Autodesk Inventor part; units mm, degrees
ref_plane "Work Plane1" through (0, 0, 0) normal (0.6427876, -0.7660444, 0) x (0, 0, -1)
ref_plane "Work Plane2" through (0, 14.3, -20) normal (-0.6427876, 0.7660444, 0) x (0, 0, -1)
ref_plane "YZ Plane" through (0, 0, 0) normal (1, 0, 0) x (0, 1, 0)
sketch "Sketch1" plane through (0, 0, 0) normal (0, 1, 0) x (-1, 0, 0)
  circle A0 centre (0, 0) radius 5.075
  circle A1 centre (0, 0) radius 20
  line L0 (1.5, -3.825) -> (-1.5, -3.825)
  line L1 (-1.5, -3.825) -> (-1.5, -6.325)
  line L2 (-1.5, -6.325) -> (1.5, -6.325)
  line L3 (1.5, -6.325) -> (1.5, -3.825)
  line L4 (1.5, -3.825) -> (-1.5, -6.325) construction
  line L5 (-1.5, -3.825) -> (1.5, -6.325) construction
  circle A2 centre (0, 0) radius 2.5
  circle A3 centre (0, 0) radius 8.754
  point P0 (0, -5.075)
  point P1 (-1.5, -4.8483)
  point P2 (1.5, -4.8483)
  dimension "d0" = 10.15
  dimension "d1" = 40
  dimension "d2" = 1.25
  dimension "d3" = 3
  dimension "d17" = 5
extrude "Extrusion1" add sketch "Sketch1" along normal blind 14.3 contours A1 | A3
sketch "Sketch2" plane through (0, 0, 0) normal (1, 0, 0) x (0, 1, 0)
  line L0 (0, 0) -> (14.3, 0)
  line L1 (14.3, 0) -> (14.3, -20)
  line L2 (14.3, -20) -> (0, -20) construction
  line L3 (0, -20) -> (0, 0)
  line L4 (0, -20) -> (14.3, -20) construction
  line L5 (14.3, -20) -> (14.3, -20.0661)
  line L6 (0, -20) -> (14.3, -20)
  circle A0 centre (7.15, -20) radius 2.5
  line L7 (9.65, -20) -> (4.65, -20)
  line L8 (4.65, -20) -> (4.65, -28)
  line L9 (4.65, -28) -> (9.65, -28)
  line L10 (9.65, -28) -> (9.65, -20)
  line L11 (14.3, -20) -> (0, -20)
  line L12 (0, -20) -> (0, -28)
  line L13 (0, -28) -> (14.3, -28)
  line L14 (14.3, -28) -> (14.3, -20)
  point P0 (14.3, -20)
  point P1 (14.3, -20)
  dimension "d22" = 5
  dimension "d7" = 20
  dimension "d10" = 14.3
  dimension "d23" = 8
  dimension "d31" = 8
  dimension "d41" = 14.3
  dimension "d42" = 5
revolve "Revolution1" add sketch "Sketch2" angle 360 about axis through (0, 0, 0) along (0, 1, 0) contours L6 L8 L13 L12 | L5 L14 L13 L10 L6
extrude "Extrusion3" add sketch "Sketch1" against normal blind 2 contours A0 L3 L0 L1 | L1 L0 L3 A0 | A0 L3 L2 L1 | A3
revolve "Revolution4" cut sketch "Sketch2" angle 360 about axis through (0, 0, 0) along (0, 1, 0) picked at (7.2504, -19.1727) contours A0 L6
sketch "Sketch3" plane through (0, 0, 0) normal (0, -1, 0) x (1, 0, 0)
  line L0 (0, 0) -> (0, -22)
  dimension "d25" = 22
ref_plane "Work Plane1" through (0, 0, 0) normal (0.6427876, -0.7660444, 0) x (0, 0, -1)
sketch "Sketch4" plane through (0, 0, 0) normal (0.6427876, -0.7660444, 0) x (0, 0, -1)
  ellipse E0 centre (0, 2.7318) end of major axis (22, 2.7318) minor radius 16.853
  line L0 (0, 0) -> (22, 0)
  circle A0 centre (22, 0) radius 3.75
  dimension "d27" = 22
  dimension "d28" = 7.5
extrude "Extrusion4" cut sketch "Sketch4" against normal blind 9 contours E0 L0 A0 | E0 A0 | E0 A0 L0 picked at (24.3646, -0.3075)
extrude "Extrusion5" cut sketch "Sketch4" along normal blind 7 contours E0 L0 A0 | E0 A0 | E0 A0 L0 picked at (24.3646, -0.3075)
ref_plane "Work Plane2" through (0, 14.3, -20) normal (-0.6427876, 0.7660444, 0) x (0, 0, -1)
sketch "Sketch5" plane through (0, 14.3, -20) normal (-0.6427876, 0.7660444, 0) x (0, 0, -1)
  ellipse E0 centre (-20, 0) end of major axis (-25.075, 0) minor radius 3.8877 (-15.1517, 1.1491) -> (-15.1517, -1.1491) ccw
  line L0 (-20, 0) -> (-42, 0)
  circle A0 centre (-42, 0) radius 3.75
  point P0 (-20, 9.1919)
  dimension "d35" = 22
  dimension "d36" = 7.5
extrude "Extrusion6" cut sketch "Sketch5" against normal blind 9
extrude "Extrusion7" cut sketch "Sketch5" along normal blind 8
extrude "Extrusion8" cut sketch "Sketch1" along normal through all contours A0 L3 L0 L1 | L1 L0 L3 A0 | A0 L3 L2 L1
sketch "Sketch6" plane through (0, 14.3, 0) normal (0, 1, 0) x (1, 0, 0)
  circle A0 centre (0, 0) radius 15
  circle A1 centre (0, 0) radius 35.6972
  dimension "d45" = 30
extrude "Extrusion9" cut sketch "Sketch6" against normal blind 2.5
sketch "Sketch7" plane through (0, 0, 0) normal (0, -1, 0) x (1, 0, 0)
  circle A0 centre (0, 0) radius 2.5
  circle A1 centre (0, 0) radius 20
  line L0 (24, -7.5) -> (-24, -7.5)
  line L1 (-24, -7.5) -> (-24, 7.5)
  line L2 (-24, 7.5) -> (24, 7.5)
  line L3 (24, 7.5) -> (24, -7.5)
  line L4 (24, -7.5) -> (-24, 7.5) construction
  line L5 (-24, -7.5) -> (24, 7.5) construction
  circle A2 centre (0, 0) radius 11
  circle A3 centre (20, 0) radius 1.9
  circle A4 centre (-20, 0) radius 1.9
  dimension "d48" = 40
  dimension "d49" = 48
  dimension "d50" = 15
  dimension "d51" = 22
  dimension "d52" = 3.8
  dimension "d53" = 3.8
extrude "Extrusion10" cut sketch "Sketch7" against normal blind 4 contours A1 A3 | A1 A3 | A4 A1 | A1 A4
properties part number "spool_temp"
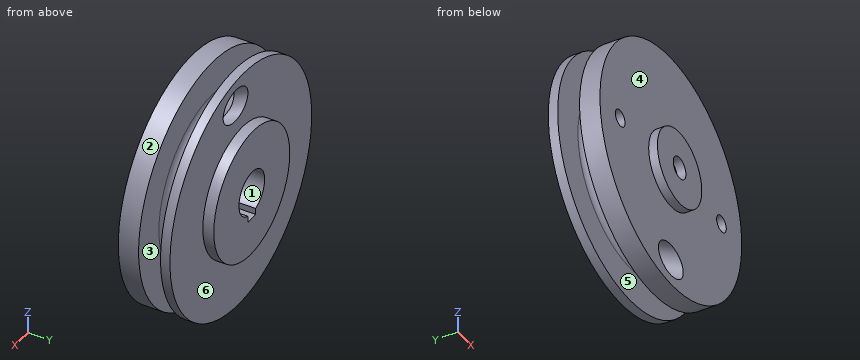
Check sheet for the modelled part. Datum: model origin and axes. Units: mm. Face numbers are marked on the shaded views. A direction names the side the tool comes from. Give positions to 0.01 mm unless a question says otherwise; leave off trailing zeros. Order: outer loops, then holes, each group sorted by start corner. A loop starts at its lowest first (then second) coordinate and runs counter-clockwise, first axis right, second up. Notation, with made-up numbers: (20.5, 24.5) -> (46.5, 24.5) arc R13 ccw to (46.5, 32.5) -> close; hole circle Ø6 at (72, 70). An arc over 180 degrees is marked (long way). Use CSV: the item, a comma, the result in double quotes. Start each with the question number.
1) Sectioned sample at A-A, the plane z = -22. Record the boundary of the cut face in (x, y), plus the area to 3 significant figures.
2) Set-up check for the marked faces 4, 5 and 6: record each of +Z, -Z, +X, -X, +Y, -Y from which the full face is reachable in a straight line by a thin tool's end or side.
3) Sectioned sample at C-C, the plane y = 0.75. Give the number of separate pieces and of enclosed holes in the cut face, plus the area to 3 significant figures.
4) Mould release check, pull along X, two halves, no side actions. Record for the marked faces 1, 2 and 3: released by +X, released by -X, zero draft, split by the parting line, or undercut.
5) Go/stop test with flat-tipped pins: P1, Ø1.9, axis at x = 20.5, z = 0.5, coming from the -Y side; P2, Ø0.7, axis at y = 7, z = -5.5, coming from the -X side; P3, Ø10, axis at x = -19.5, z = 7.5, coming from the -Y side; P4, Ø4.5, axis at x = 0, z = 0, coming from the -Y side. Record where each tip stops, or that it passes through.
6) Material ranges on line 1 (X direction, y = 2.5, z = 0) (3 decimals); line 2 (Y direction, x = 6.5, z = -25.5); line 3 (Z direction, x = 0, y = -1.3), recorded low to high. Write a range as from..to.
7) Sectioned sample at B-B, the plane x = 23. Record the boundary of the cut face in (y, z).
Recorded:
1,outline,"(-17.32, 0) -> (-4.9, 0) -> (-8.66, 4.49) -> (-8.46, 4.65) -> (-17.32, 4.65) -> close; (-17.32, 9.65) -> (17.32, 9.65) -> (17.32, 11.8) -> (-17.32, 11.8) -> close; (0.99, 4.65) -> (4.9, 0) -> (17.32, 0) -> (17.32, 4.65) -> close"
1,area,"190 mm2"
2,face 4,"-Y"
2,face 5,"none"
2,face 6,"+Y"
3,separate pieces,"1"
3,enclosed holes,"4"
3,area,"2,300 mm2"
4,face 1,"undercut"
4,face 2,"split by the parting line"
4,face 3,"zero draft"
5,P1,"y = 4"
5,P2,"x = -16.73"
5,P3,"y = 0"
5,P4,"through"
6,line 1,"-28..-21.9, -18.1..-5.075, 5.075..18.1, 21.9..28"
6,line 2,"0..4.65, 9.65..11.8"
6,line 3,"-8.75..-2.5, 2.5..8.75"
7,outline,"(0, -15.97) -> (4.65, -15.97) -> (4.65, 15.97) -> (0, 15.97) -> close; (9.65, -15.97) -> (11.8, -15.97) -> (11.8, 15.97) -> (9.65, 15.97) -> close"
